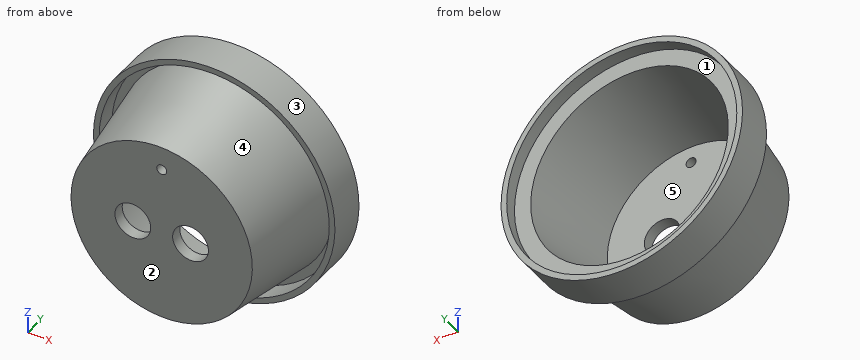
from build123d import *

# Parameters (mm, degrees)
SKETCH2_R          = 8.001
SKETCH2_R_2        = 2.2225
CUT_EXTRUDE1_DEPTH = 91.48908463


with BuildPart() as part:
    # Sketch1 → Revolve1 (revolve)
    with BuildSketch(Plane.XY, mode=Mode.PRIVATE) as revolve1_sk:
        Polygon((37.465, 4.32701069), (44.163455703, 47.50701069), (51.435, 47.50701069), (51.435, 52.924059852), (53.975, 52.924059852), (53.975, 46.574059852), (53.975, 36.07701069), (51.435, 36.07701069), (51.435, 44.96701069), (47.625, 44.96701069), (40.532517491, -0.75298931), (0, -0.75298931), (0, 4.32701069), align=None)
    revolve(revolve1_sk.sketch.rotate(Axis((0, 0, 0), (0, 1, 0)), 90), axis=Axis((0, 0, 0), (0, 1, 0)))

    # Sketch2 → Cut-Extrude1 (cut, through all)
    with BuildSketch(Plane(origin=(0, 4.32701069, 0), x_dir=(1, 0, 0), z_dir=(0, 1, 0))):
        with Locations(Location((-12.89685, 0, 0), (0, 0, 270))):
            Circle(SKETCH2_R)
        with Locations(Location((12.89685, 0, 0), (0, 0, 270))):
            Circle(SKETCH2_R)
        with Locations(Location((0, -29.968876042, 0), (0, 0, 270))):
            Circle(SKETCH2_R_2)
    extrude(amount=-CUT_EXTRUDE1_DEPTH, mode=Mode.SUBTRACT)


solid = part.part
Build history of the part. All positions in model axes, mm. Face numbers are marked on the shaded views. A direction names the side the tool comes from. Coordinates: 2 decimals unless noted, no trailing zeros. Write each loop counter-clockwise with the first axis right and the second up, starting at its lowest first coordinate (ties: lowest second). Pieces come first, ordered by that corner, then holes.
(1) Cut at C-C on y = 40. List the corners of the cut face in (x, z) (3 decimals), and give its area (3 significant figures).
(2) Mould opens along X. For the marked faces 1, 2 and 3 say: pulls with the +X half, pulls with the -X half, needs draft (parallel to the pull), parting line crosses it, or undercut.
(3) 3-axis set-ups, long thin cutter, end or side, ignore diameter. For the marked faces 4 and 5: which of +Z, -Z, +X, -X, +Y, -Y reach the whole face in a straight line?
(4) Cut at D-D on y = 13.5. List the corners of the cut face in (x, z).
(5) Cut at B-B on x = 0. List the corners of the cut face in (y, z) (3 decimals), and give its area (3 significant figures).
(6) Cut at A-A on z = 0. List the corners of the cut face in (x, y) (3 decimals).
(7) Drill centre lines: line 1 (Z direction, x = -17, y = 36.5); line 2 (Y direction, x = 28.5, z = 43.5); line 3 (X direction, y = 37, z = 0) (3 decimals). Where is each one in solid material? Low to high.
(8) Pin check, flat tips, straight feed: pin 1 Ø4 at (y, z) = (19.5, 3) entering from +X; pin 2 Ø1 at (x, y) = (17.5, 16.5) entering from +Z; pin 3 Ø3 at (y, z) = (29, 40) entering from -X. Stop position of each tip, or through.
Working result:
1. outline: circle Ø107.95 at (0, 0); circle Ø93.709 at (0, 0); hole circle Ø102.87 at (0, 0); hole circle Ø85.998 at (0, 0)
1. area: 1,930 mm2
2. face 1: undercut
2. face 2: needs draft
2. face 3: parting line crosses it
3. face 4: -Y
3. face 5: +Y
4. outline: circle Ø85.49 at (0, 0); hole circle Ø77.78 at (0, 0)
5. outline: (-0.753, -40.533) - (44.967, -47.625) - (44.967, -51.435) - (36.077, -51.435) - (36.077, -53.975) - (52.924, -53.975) - (52.924, -51.435) - (47.507, -51.435) - (47.507, -44.163) - (4.327, -37.465) - (4.327, 27.746) - (-0.753, 27.746) - close; (-0.753, 32.191) - (4.327, 32.191) - (4.327, 37.465) - (47.507, 44.163) - (47.507, 51.435) - (52.924, 51.435) - (52.924, 53.975) - (36.077, 53.975) - (36.077, 51.435) - (44.967, 51.435) - (44.967, 47.625) - (-0.753, 40.533) - close
5. area: 830 mm2
6. outline: (-53.975, 36.077) - (-51.435, 36.077) - (-51.435, 44.967) - (-47.625, 44.967) - (-40.533, -0.753) - (-20.898, -0.753) - (-20.898, 4.327) - (-37.465, 4.327) - (-44.163, 47.507) - (-51.435, 47.507) - (-51.435, 52.924) - (-53.975, 52.924) - close; (-4.896, -0.753) - (4.896, -0.753) - (4.896, 4.327) - (-4.896, 4.327) - close; (20.898, -0.753) - (40.533, -0.753) - (47.625, 44.967) - (51.435, 44.967) - (51.435, 36.077) - (53.975, 36.077) - (53.975, 52.924) - (51.435, 52.924) - (51.435, 47.507) - (44.163, 47.507) - (37.465, 4.327) - (20.898, 4.327) - close
7. line 1: z = -51.23 to -48.54, -43.08 to -38.9, 38.9 to 43.08, 48.54 to 51.23
7. line 2: y = 36.08 to 52.92
7. line 3: x = -53.975 to -51.435, -46.389 to -42.534, 42.534 to 46.389, 51.435 to 53.975
8. pin 1: stops at x = 43.9
8. pin 2: stops at z = 39.74
8. pin 3: stops at x = -23.62
